```python
from build123d import *

# Parameters (mm, degrees)
SKETCH_1_R      = 5
EXTRUDE_1_DEPTH = 10
FILLET_1_R      = 1


with BuildPart() as part:
    # Эскиз1 → Вытянуть1 (new body)
    with BuildSketch(Plane.XY):
        Polygon((9.732299753, 2.298334508), (2.875733806, 9.577586078), (-6.856565947, 7.27925157), (-9.732299753, -2.298334508), (-2.875733806, -9.577586078), (6.856565947, -7.27925157), align=None)
        Circle(SKETCH_1_R, mode=Mode.SUBTRACT)
    extrude(amount=EXTRUDE_1_DEPTH)

    # Скругление1
    fillet_1_edges = [part.edges().sort_by_distance(p)[0] for p in [
        (-1.99041607, 8.428418824, 10),
        (-8.29443285, 2.490458531, 10),
        (-6.30401678, -5.937960293, 10),
        (1.99041607, -8.428418824, 10),
        (8.29443285, -2.490458531, 10),
        (1.99041607, -8.428418824, 0),
        (-6.30401678, -5.937960293, 0),
        (-8.29443285, 2.490458531, 0),
        (6.30401678, 5.937960293, 10),
        (-1.99041607, 8.428418824, 0),
        (6.30401678, 5.937960293, 0),
        (8.29443285, -2.490458531, 0),
    ]]
    fillet(fillet_1_edges, radius=FILLET_1_R)


solid = part.part
```
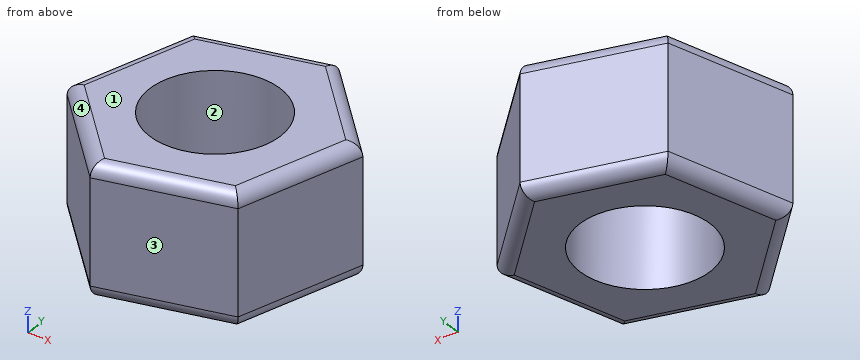
Read the model definition and answer for the solid it produces. Units are mm, in the model's axes. Face numbers are marked on the shaded views. Round coordinates to 2 decimals unless told otherwise and drop trailing zeros. Write each loop counter-clockwise with the first axis right and the second up, starting at its lowest first coordinate (ties: lowest second). Pieces come first, ordered by that corner, then holes. Notation, with made-up numbers: M 71,24 L 126,24 A23 ccw 126,49 Z; hole C 45,64.5 d1. An arc over 180 degrees is marked long. One line per item, written item: value.
Q1. For a pull along X with two mould halves and no side action, classify the marked faces 1, 2, 3 and 4 as +X half, -X half, draft (parallel to the pull), parting line (faces both ways), or undercut.
Data:
face 1: draft
face 2: undercut
face 3: +X half
face 4: -X half
Q2. Flat-ended cylindrical pins translate along their axes: pin 1 Ø9 at (x, y) = (0, 0) entering from -Z; pin 2 Ø5 at (y, z) = (1, 8.5) entering from -X; pin 3 Ø4 at (y, z) = (-3.5, 6.5) entering from +X. Find the tip coordinate at first contact, or state that the pin passes through.
Data:
pin 1: through
pin 2: x = -9.49
pin 3: x = 8.59
Q3. Straight lines are drawn through the part: line 1 (Y direction, x = 0, z = 5.25); line 2 (X direction, y = -0.5, z = 3.5); line 3 (Y direction, x = -1, z = 8.25). For each, find the intervals that lie inside material, in ascending order. Write a range as [from, to].
Data:
line 1: [-8.9, -5], [5, 8.9]
line 2: [-9.19, -4.97], [4.97, 8.89]
line 3: [-9.13, -4.9], [4.9, 8.66]
Q4. Find section A-A on z = 6.25. Write down the section's boundary in (x, y), plus the area to 3 significant figures.
Data:
outline: M -9.73,-2.3 L -2.88,-9.58 L 6.86,-7.28 L 9.73,2.3 L 2.88,9.58 L -6.86,7.28 Z; hole C 0,0 d10
area: 181 mm2
